The listing builds one solid part. Answer for the finished solid, in the listing's coordinates (mm). Face numbers are marked on the shaded views. A direction names the side the tool comes from. Round coordinates to 2 decimals unless told otherwise and drop trailing zeros. Order: outer loops, then holes, each group sorted by start corner. A loop starts at its lowest first (then second) coordinate and runs counter-clockwise, first axis right, second up. Notation, with made-up numbers: (17.5, 76) - (70.5, 76) arc R20 ccw to (70.5, 100) - close; hole circle Ø11 at (53, 4). An arc over 180 degrees is marked (long way). Write item = value, one per line.
from build123d import *

# Parameters (mm, degrees)
F0_R     = 3.25
F1_DEPTH = 7
F2_DEPTH = 10
F3_COUNT = 3


with BuildPart() as f1:
    # F0 (on Front) → F1 (new body)
    with BuildSketch(Plane.XZ):
        with BuildLine():
            Line((17.3205080757, 10), (28.5788383249, 16.5))
            ThreePointArc((28.5788383249, 16.5), (0, 33), (-28.5788383249, 16.5))
            Line((-28.5788383249, 16.5), (-17.3205080757, 10))
            ThreePointArc((-17.3205080757, 10), (0, 20), (17.3205080757, 10))
        make_face()
        with Locations((0, 25.8179008961)):
            Circle(F0_R, mode=Mode.SUBTRACT)
    extrude(amount=F1_DEPTH)

    # F0 (on Front) → F2 (join)
    with BuildSketch(Plane.XZ):
        with BuildLine():
            Line((8.6602540378, 5), (17.3205080757, 10))
            ThreePointArc((17.3205080757, 10), (0, 20), (-17.3205080757, 10))
            Line((-17.3205080757, 10), (-8.6602540378, 5))
            ThreePointArc((-8.6602540378, 5), (0, 10), (8.6602540378, 5))
        make_face()
    extrude(amount=F2_DEPTH)

    # F3: F1 ×3 about axis
    f3_axis = Axis((0, 0, 0), (0, -1, 0))


with BuildPart() as f1_1:
    add(f1.part)
    for i in range(1, F3_COUNT):
        add(f1.part.rotate(f3_axis, i * 360 / F3_COUNT))


solid = f1_1.part
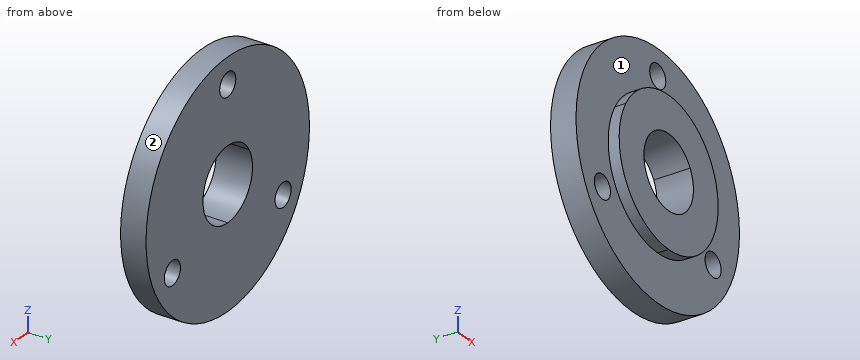
Q1. Section A-A on z = 0 is taken. Determine the outline of the cut face in (x, y).
Model answer:
outline = (-33, -7) - (-20, -7) - (-20, -10) - (-10, -10) - (-10, 0) - (-33, 0) - close; (10, -10) - (20, -10) - (20, -7) - (33, -7) - (33, 0) - (10, 0) - close
Q2. Find the intervals of material crossed by line 1 (Z direction, x = -0.5, y = -1.75); line 2 (Y direction, x = 14.5, z = 16); line 3 (X direction, y = -4.5, z = 6.5), in increasing order. Write a range as from..to.
Model answer:
line_1 = -33..-9.99, 9.99..22.61, 29.03..33
line_2 = -7..0
line_3 = -32.35..-7.6, 7.6..32.35
Q3. Section D-D on y = -5.25 is taken. Determine the outline of the cut face in (x, z).
Model answer:
outline = circle Ø66 at (0, 0); hole circle Ø6.5 at (-22.36, -12.91); hole circle Ø20 at (0, 0); hole circle Ø6.5 at (0, 25.82); hole circle Ø6.5 at (22.36, -12.91)
Q4. Section C-C on x = -7 is taken. Determine the outline of the cut face in (y, z) (3 decimals).
Model answer:
outline = (-10, -18.735) - (-7, -18.735) - (-7, -32.249) - (0, -32.249) - (0, -7.141) - (-10, -7.141) - close; (-10, 7.141) - (0, 7.141) - (0, 32.249) - (-7, 32.249) - (-7, 18.735) - (-10, 18.735) - close
Q5. Flat-ended cylindrical pins translate along their axes: P1, Ø6, axis at y = -2, z = 18.5, coming from the -X side; P2, Ø10.5, axis at x = -22.36, z = -12.91, coming from the +Y side; P3, Ø4, axis at y = -1.5, z = -5, coming from the +X side; P4, Ø6, axis at y = -5, z = 9.5, coming from the -X side. Find the tip coordinate at first contact, or state that the pin passes through.
Model answer:
P1 = -29.13
P2 = 0
P3 = 32.86
P4 = -32.35
Q6. Section B-B on y = -8.75 is taken. Determine the outline of the cut face in (x, z), then the cut area to 3 significant figures.
Model answer:
outline = circle Ø40 at (0, 0); hole circle Ø20 at (0, 0)
area = 942 mm^2
Q7. For the marked faces 1 and 2, determine the directions among +Z, -Z, +X, -X, +Y, -Y from which every point of the face is accessible in a straight line to the end or side of a thin tool.
Model answer:
face_1 = -Y
face_2 = +Y, -Y
